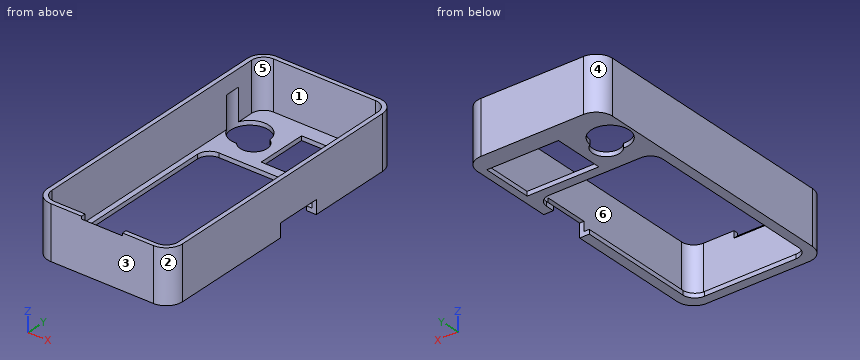
from build123d import *

# Parameters (mm, degrees)
BOSS_EXTRUDE1_DEPTH = 6.999999996
SKETCH2_R           = 7.875521796
BOSS_EXTRUDE2_DEPTH = 15.032422661
SKETCH3_R           = 5.636
SKETCH3_W           = 29.8
SKETCH3_H           = 21.2
CUT_EXTRUDE1_DEPTH  = 6.88
CUT_EXTRUDE2_DEPTH  = 13.232422661
SKETCH5_W           = 6.5
SKETCH5_H           = 18.860946171
CUT_EXTRUDE3_DEPTH  = 6.88
CUT_EXTRUDE4_DEPTH  = 8.52


with BuildPart() as part:
    # Sketch1 → Boss-Extrude1 (new body)
    with BuildSketch(Plane.XY):
        with BuildLine():
            Line((64.993664433, 62.013874967), (64.993664433, 166.948874967))
            ThreePointArc((64.993664433, 166.948874967), (63.001990545, 171.757201079), (58.193664433, 173.748874967))
            Line((58.193664433, 173.748874967), (15.615664433, 173.748874967))
            ThreePointArc((15.615664433, 173.748874967), (10.807338321, 171.757201079), (8.815664433, 166.948874967))
            Line((8.815664433, 166.948874967), (8.815664433, 62.013874967))
            ThreePointArc((8.815664433, 62.013874967), (10.807338321, 57.205548855), (15.615664433, 55.213874967))
            Line((15.615664433, 55.213874967), (58.193664433, 55.213874967))
            ThreePointArc((58.193664433, 55.213874967), (63.001990545, 57.205548855), (64.993664433, 62.013874967))
        make_face()
        with BuildLine():
            Line((63.193664433, 62.013874967), (63.193664433, 166.948874967))
            ThreePointArc((63.193664433, 166.948874967), (61.729198339, 170.484408873), (58.193664433, 171.948874967))
            Line((58.193664433, 171.948874967), (15.615664433, 171.948874967))
            ThreePointArc((15.615664433, 171.948874967), (12.080130527, 170.484408873), (10.615664433, 166.948874967))
            Line((10.615664433, 166.948874967), (10.615664433, 62.013874967))
            ThreePointArc((10.615664433, 62.013874967), (12.080130527, 58.478341061), (15.615664433, 57.013874967))
            Line((15.615664433, 57.013874967), (58.193664433, 57.013874967))
            ThreePointArc((58.193664433, 57.013874967), (61.729198339, 58.478341061), (63.193664433, 62.013874967))
        make_face(mode=Mode.SUBTRACT)
    extrude(amount=-BOSS_EXTRUDE1_DEPTH)

    # Sketch2 → Boss-Extrude2 (add)
    with BuildSketch(Plane(origin=(0, 0, -6.999999996), x_dir=(-1, 0, 0), z_dir=(0, 0, -1))):
        with BuildLine():
            Line((-58.193664433, 55.213874967), (-15.615664433, 55.213874967))
            ThreePointArc((-15.615664433, 55.213874967), (-10.807338321, 57.205548855), (-8.815664433, 62.013874967))
            Line((-8.815664433, 62.013874967), (-8.815664433, 166.948874967))
            ThreePointArc((-8.815664433, 166.948874967), (-10.807338321, 171.757201079), (-15.615664433, 173.748874967))
            Line((-15.615664433, 173.748874967), (-58.193664433, 173.748874967))
            ThreePointArc((-58.193664433, 173.748874967), (-63.001990545, 171.757201079), (-64.993664433, 166.948874967))
            Line((-64.993664433, 166.948874967), (-64.993664433, 62.013874967))
            ThreePointArc((-64.993664433, 62.013874967), (-63.001990545, 57.205548855), (-58.193664433, 55.213874967))
        make_face()
        with Locations(Location((-17.816098985, 156.86861317, 0), (0, 0, 90))):
            Circle(SKETCH2_R, mode=Mode.SUBTRACT)
    extrude(amount=BOSS_EXTRUDE2_DEPTH)

    # Sketch3 → Cut-Extrude1 (cut)
    with BuildSketch(Plane(origin=(0, 0, -22.032422657), x_dir=(-1, 0, 0), z_dir=(0, 0, -1))):
        with Locations((-22.802237874, 152.631613686)):
            Circle(SKETCH3_R)
        with BuildLine():
            Line((-60.993664433, 135.686808525), (-60.993664433, 64.213874967))
            ThreePointArc((-60.993664433, 64.213874967), (-59.529198339, 60.678341061), (-55.993664433, 59.213874967))
            Line((-55.993664433, 59.213874967), (-17.815664433, 59.213874967))
            ThreePointArc((-17.815664433, 59.213874967), (-14.280130527, 60.678341061), (-12.815664433, 64.213874967))
            Line((-12.815664433, 64.213874967), (-12.815664433, 135.686808525))
            ThreePointArc((-12.815664433, 135.686808525), (-14.280130527, 139.222342431), (-17.815664433, 140.686808525))
            Line((-17.815664433, 140.686808525), (-55.993664433, 140.686808525))
            ThreePointArc((-55.993664433, 140.686808525), (-59.529198339, 139.222342431), (-60.993664433, 135.686808525))
        make_face()
        with Locations((-47.079251594, 155.286808525)):
            Rectangle(SKETCH3_W, SKETCH3_H)
    extrude(amount=-CUT_EXTRUDE1_DEPTH, mode=Mode.SUBTRACT)

    # Sketch4 → Cut-Extrude2 (cut)
    with BuildSketch(Plane.XY.offset(-6.999999996)):
        with BuildLine():
            Line((15.615664433, 57.013874967), (58.193664433, 57.013874967))
            ThreePointArc((58.193664433, 57.013874967), (61.729198339, 58.478341061), (63.193664433, 62.013874967))
            Line((63.193664433, 62.013874967), (63.193664433, 166.948874967))
            ThreePointArc((63.193664433, 166.948874967), (61.729198339, 170.484408873), (58.193664433, 171.948874967))
            Line((58.193664433, 171.948874967), (15.615664433, 171.948874967))
            ThreePointArc((15.615664433, 171.948874967), (12.080130527, 170.484408873), (10.615664433, 166.948874967))
            Line((10.615664433, 166.948874967), (10.615664433, 160.058846048))
            ThreePointArc((10.615664433, 160.058846048), (25.691620781, 156.86861317), (10.615664433, 153.678380292))
            Line((10.615664433, 153.678380292), (10.615664433, 62.013874967))
            ThreePointArc((10.615664433, 62.013874967), (12.080130527, 58.478341061), (15.615664433, 57.013874967))
        make_face()
    extrude(amount=-CUT_EXTRUDE2_DEPTH, mode=Mode.SUBTRACT)

    # Sketch5 → Cut-Extrude3 (cut)
    with BuildSketch(Plane(origin=(64.993664433, 0, 0), x_dir=(0, 0, -1), z_dir=(1, 0, 0))):
        with Locations((19.582422658, 122.741984607)):
            Rectangle(SKETCH5_W, SKETCH5_H)
    extrude(amount=-CUT_EXTRUDE3_DEPTH, mode=Mode.SUBTRACT)

    # Sketch6 → Cut-Extrude4 (cut, symmetric)
    with BuildSketch(Plane.ZY.offset(-36.904664433)):
        Polygon((0, 57.013874967), (-2.853568486, 57.013874967), (-1.108049312, 55.213874967), (0, 55.213874967), align=None)
    extrude(amount=CUT_EXTRUDE4_DEPTH, both=True, mode=Mode.SUBTRACT)


solid = part.part
Design review of the part built by this model. Coordinates are the model's own, in mm. Face numbers are marked on the shaded views. A direction names the side the tool comes from. Give positions to 0.01 mm unless a question says otherwise; leave off trailing zeros. Order: outer loops, then holes, each group sorted by start corner. A loop starts at its lowest first (then second) coordinate and runs counter-clockwise, first axis right, second up. Notation, with made-up numbers: (68.25, -6.5) - (105.25, -6.5) arc R18 cw to (105.25, 16.5) - close; hole circle Ø5 at (40, 86.25). An arc over 180 degrees is marked (long way). Write item = value, one per line. Start each with the question number.
Q1. We need section B-B on y = 68. State the section outline as (x, z) points.
Q2. We need section C-C on z = -12.5. State the section outline as (x, y) points.
Q3. To check wall thickness, follow L1, parallel to X at y = 97, z = -11.5; L2, parallel to Y at x = 46.5, z = -13; L3, parallel to Z at x = 22, y = 146. State the ranges of each line that lie inside material, in increasing order. Write a range as from..to.
Q4. Mouldability with a two-part tool opening along X and no side actions: class the marked faces 3, 4, 5 and 6 as released by +X, released by -X, zero draft, split by the parting line, or undercut.
Q5. We need section D-D on y = 142.5. State the section outline as (x, z) points.
Q6. Clearance check with flat-ended pins moving along their axes: pin 1 Ø1.4 at (x, y) = (64, 119.5) entering from -Z; pin 2 Ø1.2 at (x, z) = (62, -20.5) entering from -Y; pin 3 Ø18 at (x, y) = (22.8, 152.63) entering from +Z. State where each tip first meets the part, or that it passes through.
Q7. Tool access review of the marked faces 1 and 2: name each direction out of +Z, -Z, +X, -X, +Y, -Y from which nothing blocks a thin tool from reaching the whole face with its end or side.
Q8. We need section A-A on x = 50. State the section outline as (y, z) points, plus the area to 3 significant figures.
Working result:
q1.outline = (8.82, -22.03) - (12.82, -22.03) - (12.82, -20.23) - (10.62, -20.23) - (10.62, 0) - (8.82, 0) - close; (60.99, -22.03) - (64.99, -22.03) - (64.99, 0) - (63.19, 0) - (63.19, -20.23) - (60.99, -20.23) - close
q2.outline = (8.82, 62.01) arc R6.8 ccw to (15.62, 55.21) - (58.19, 55.21) arc R6.8 ccw to (64.99, 62.01) - (64.99, 166.95) arc R6.8 ccw to (58.19, 173.75) - (15.62, 173.75) arc R6.8 ccw to (8.82, 166.95) - close; hole (10.62, 62.01) arc R5 ccw to (15.62, 57.01) - (58.19, 57.01) arc R5 ccw to (63.19, 62.01) - (63.19, 166.95) arc R5 ccw to (58.19, 171.95) - (15.62, 171.95) arc R5 ccw to (10.62, 166.95) - (10.62, 160.06) arc R7.88 ccw to (10.62, 153.68) - close
q3.L1 = 8.82..10.62, 63.19..64.99
q3.L2 = 55.21..57.01, 171.95..173.75
q3.L3 = -22.03..-20.23
q4.face_3 = zero draft
q4.face_4 = released by -X
q4.face_5 = undercut
q4.face_6 = undercut
q5.outline = (8.82, -22.03) - (64.99, -22.03) - (64.99, 0) - (63.19, 0) - (63.19, -20.23) - (10.62, -20.23) - (10.62, 0) - (8.82, 0) - close
q6.pin_1 = -16.33
q6.pin_2 = 56.02
q6.pin_3 = -20.23
q7.face_1 = +Z
q7.face_2 = +Z, -Z, +X, -Y
q8.outline = (55.21, -22.03) - (59.21, -22.03) - (59.21, -20.23) - (57.01, -20.23) - (57.01, 0) - (55.21, 0) - close; (140.69, -22.03) - (144.69, -22.03) - (144.69, -20.23) - (140.69, -20.23) - close; (165.89, -22.03) - (173.75, -22.03) - (173.75, 0) - (171.95, 0) - (171.95, -20.23) - (165.89, -20.23) - close
q8.area = 101 mm²
